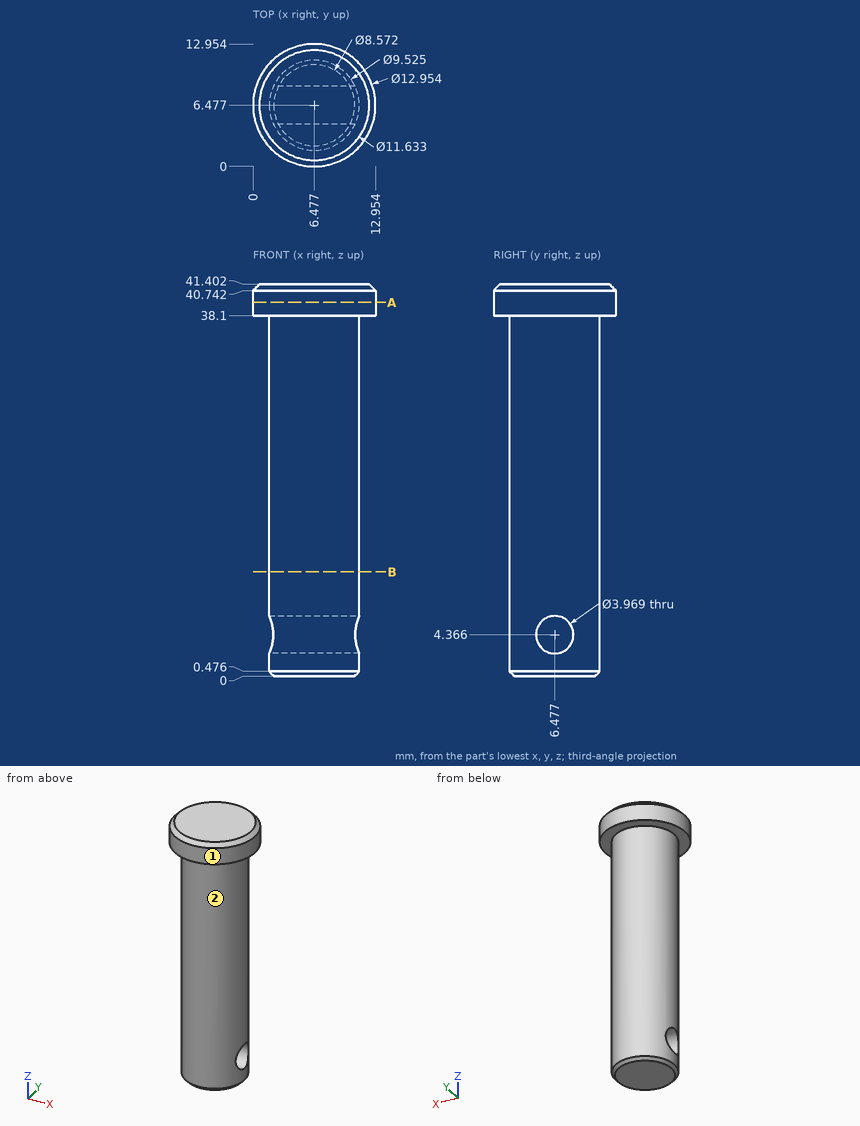
Answer from the drawing. Dimensions are ordinates in mm from the lowest x, y and z of the part. A direction names the side the tool comes from. Coordinates: 2 decimals unless noted, no trailing zeros. Loops run counter-clockwise (first coordinate to the right, second up) from the corner with the lowest first, then second, coordinate; pieces in that order, holes last.
1) Section B-B (z = 11) is taken. Give the vertices of the cut face in (x, y) (1 decimal).
Results:
outline: circle Ø9.5 at (6.5, 6.5)
2) Flat-ended cylindrical pins translate along their axes: pin 1 (2 mm diameter, centred on x = 11.5, z = 5.5, fed in from +Y) (1 decimal); pin 2 (4 mm diameter, centred on y = 4.5, z = 35, fed in from -X) (1 decimal); pin 3 (6 mm diameter, centred on x = 9.5, z = 20, fed in from +Y); pin 4 (3.5 mm diameter, centred on y = 6.48, z = 4.37, fed in from +X). Find the tip coordinate at first contact, or state that the pin passes through.
Results:
pin 1: stops at y = 9
pin 2: stops at x = 1.7
pin 3: stops at y = 11.24
pin 4: passes through
3) For the marked faces 1 and 2, determine the directions among +Z, -Z, +X, -X, +Y, -Y from which every point of the face is accessible in a straight line to the end or side of a thin tool.
Results:
face 1: +Z, -Z
face 2: -Z
4) Consider probe 1 along X at (y, z) = (6.75, 35.5); probe 2 along Z at (x, y) = (11.75, 6.25); probe 3 along Z at (x, y) = (11, 5.25) (1 decimal). Determine where each line is inside the solid, lowest interval first.
Results:
probe 1: x = 1.72 to 11.23
probe 2: z = 38.1 to 41.4
probe 3: z = 0.4 to 2.8, 5.9 to 41.4
5) Section A-A (z = 39.5) is taken. Give the vertices of the cut face in (x, y) (1 decimal), plus the area to 3 significant figures.
Results:
outline: circle Ø13 at (6.5, 6.5)
area: 132 mm2
